```python
from build123d import *

# Parameters (mm, degrees)
SKETCH1_W           = 20
SKETCH1_H           = 15
BOSS_EXTRUDE1_DEPTH = 5
SKETCH2_R           = 1.5
CUT_EXTRUDE1_DEPTH  = 24.203994107
SKETCH3_R           = 4
CUT_EXTRUDE2_DEPTH  = 5


with BuildPart() as part:
    # Sketch1 → Boss-Extrude1 (new body)
    with BuildSketch(Plane(origin=(0, 0, 0), x_dir=(1, 0, 0), z_dir=(0, 1, 0))):
        with Locations((-6.983089899, -4.822749115)):
            Rectangle(SKETCH1_W, SKETCH1_H)
    extrude(amount=BOSS_EXTRUDE1_DEPTH)

    # Sketch2 → Cut-Extrude1 (cut, through all)
    with BuildSketch(Plane.XY.offset(12.322749115)):
        with Locations((-13.983089899, 2.5)):
            Circle(SKETCH2_R)
        with Locations(Location((0.016910101, 2.5, 0), (0, 0, 180))):
            Circle(SKETCH2_R)
    extrude(amount=-CUT_EXTRUDE1_DEPTH, mode=Mode.SUBTRACT)

    # Sketch3 → Cut-Extrude2 (cut)
    with BuildSketch(Plane(origin=(0, 5, 0), x_dir=(1, 0, 0), z_dir=(0, 1, 0))):
        with Locations(Location((-7.080321074, -4.822749115, 0), (0, 0, 270))):
            Circle(SKETCH3_R)
    extrude(amount=-CUT_EXTRUDE2_DEPTH, mode=Mode.SUBTRACT)


solid = part.part
```
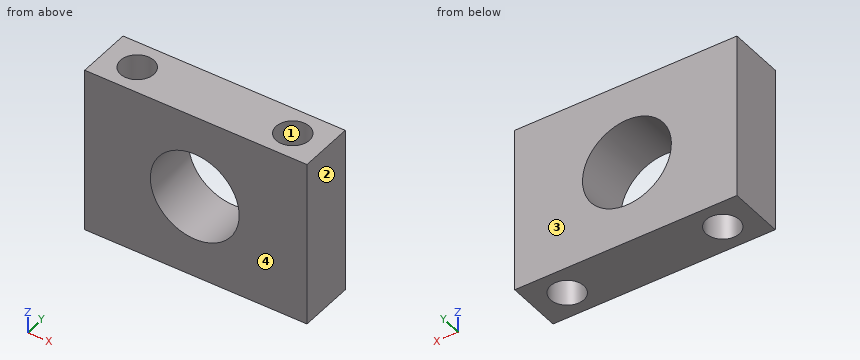
Geometry check sheet. Reference: the model listing, model coordinates, mm. Face numbers are marked on the shaded views. Coordinates: 2 decimals unless noted, no trailing zeros. Order: outer loops, then holes, each group sorted by start corner. A loop starts at its lowest first (then second) coordinate and runs counter-clockwise, first axis right, second up. Notation, with made-up numbers: (44.25, 38) - (70.25, 38) arc R7 cw to (70.25, 42) - close; hole circle Ø3 at (6, 29.25). An arc over 180 degrees is marked (long way). Answer in a Markdown table with one row per item. Add a question column.
1. Section check B-B (z = 10.25). Enter the section's corners in (x, y).
2. Section check A-A (y = 2.5). Enter the section's corners in (x, z), plus the area to 3 significant figures.
3. Material ranges on L1, parallel to X at y = 1.8, z = 5.5; L2, parallel to X at y = 3.45, z = -2; L3, parallel to Z at x = -9, y = 4.4, recorded low to high. Write a range as [from, to].
4. Draft check along Y on the marked faces 1, 2, 3 and 4. Enter one of: +Y half, -Y half, draft (parallel to the pull), parting line (faces both ways), or undercut.
5. Section check C-C (x = -6.5). Enter the section's corners in (y, z).
6. Section check D-D (z = 2.75). Enter the section's corners in (x, y).
Data:
| question | item | result |
|---|---|---|
| 1 | outline | (-16.98, 0) - (3.02, 0) - (3.02, 5) - (-16.98, 5) - close; hole circle Ø3 at (-13.98, 2.5); hole circle Ø3 at (0.02, 2.5) |
| 2 | outline | (-16.98, -2.68) - (-15.48, -2.68) - (-15.48, 12.32) - (-16.98, 12.32) - close; (-12.48, -2.68) - (-1.48, -2.68) - (-1.48, 12.32) - (-12.48, 12.32) - close; (1.52, -2.68) - (3.02, -2.68) - (3.02, 12.32) - (1.52, 12.32) - close; hole circle Ø8 at (-7.08, 4.82) |
| 2 | area | 160 mm² |
| 3 | L1 | x = [-16.98, -15.31], [-12.66, -11.02], [-3.14, -1.31], [1.34, 3.02] |
| 3 | L2 | x = [-16.98, -15.14], [-12.82, -1.14], [1.18, 3.02] |
| 3 | L3 | z = [-2.68, 1.31], [8.33, 12.32] |
| 4 | face 1 | undercut |
| 4 | face 2 | draft |
| 4 | face 3 | +Y half |
| 4 | face 4 | -Y half |
| 5 | outline | (0, -2.68) - (5, -2.68) - (5, 0.87) - (0, 0.87) - close; (0, 8.78) - (5, 8.78) - (5, 12.32) - (0, 12.32) - close |
| 6 | outline | (-16.98, 0) - (-10.5, 0) - (-10.5, 5) - (-16.98, 5) - close; (-3.66, 0) - (3.02, 0) - (3.02, 5) - (-3.66, 5) - close; hole circle Ø3 at (-13.98, 2.5); hole circle Ø3 at (0.02, 2.5) |
